Read the model definition and answer for the solid it produces. Units are mm, in the model's axes. Face numbers are marked on the shaded views. Round coordinates to 2 decimals unless told otherwise and drop trailing zeros. Write each loop counter-clockwise with the first axis right and the second up, starting at its lowest first coordinate (ties: lowest second). Pieces come first, ordered by that corner, then holes. Notation, with made-up numbers: (52.5, -20.5) - (65.5, -20.5) arc R38 cw to (65.5, 18.5) - close; hole circle Ø7 at (51, -40). An arc over 180 degrees is marked (long way). Use one line per item in the form item = value. Start each with the question number.
1) The part is cut by section A-A, the plane y = 326. Give the vertices of the cut face in (x, z) (3 decimals).
2) The part is cut by section C-C, the plane z = 211.5. Give the vertices of the cut face in (x, y) (3 decimals).
3) For a pull along X with two mould halves and no side action, classify the marked faces 1, 2 and 3 as released by +X, released by -X, zero draft, split by the parting line, or undercut.
4) Consider line 1 along X through (y, z) = (326, 202) (3 decimals); line 2 along Y through (x, z) = (172, 225) (3 decimals); line 3 along Z through (x, y) = (167.75, 326) (3 decimals). Determine where each line is inside the solid, lowest interval first. Write a range as from..to.
5) Each of these flat-tipped pins is pushed along its axis until it touches: pin 1 (1 mm diameter, centred on x = 172.5, y = 325, fed in from -Z); pin 2 (1.5 mm diameter, centred on y = 328.5, z = 221.5, fed in from -X); pin 3 (1.5 mm diameter, centred on x = 173.5, z = 220, fed in from +Y); pin 4 (2 mm diameter, centred on x = 175.5, y = 327, fed in from -Z) (3 decimals). Where does it stop, or does it pass through?
6) The part is cut by section B-B, the plane x = 165.5. Give the vertices of the cut face in (y, z) (3 decimals), plus the area to 3 significant figures.
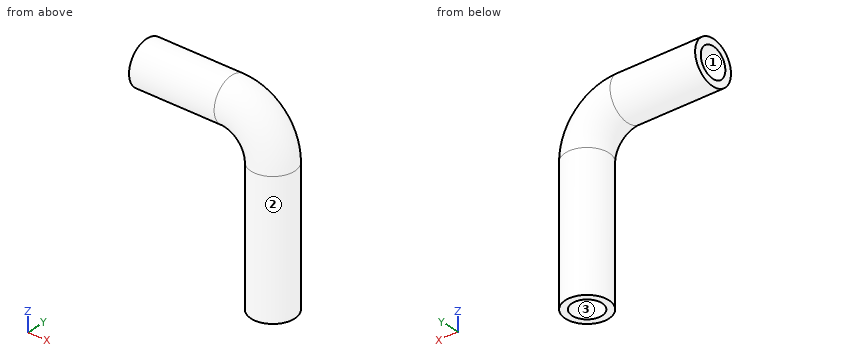
from build123d import *

# Parameters (mm, degrees)
TUBE_PROFILE_R   = 3.175
TUBE_PROFILE_R_2 = 2.175


with BuildPart() as part:
    # Tube: sweep along a curve in space
    with BuildLine() as tube_path:
        Line((182, 326, 199.5), (182, 326, 219))
        ThreePointArc((176, 326, 225), (180.242640687, 326, 223.242640687), (182, 326, 219))
        Line((176, 326, 225), (163.5, 326, 225))
    # Tube profile (on start of the path) → Tube (sweep)
    with BuildSketch(Plane(origin=(182, 326, 199.5), x_dir=(1, 0, 0), z_dir=(0, 0, 1))):
        Circle(TUBE_PROFILE_R)
        Circle(TUBE_PROFILE_R_2, mode=Mode.SUBTRACT)
    sweep(path=tube_path.line)


solid = part.part
Geometry results:
q1.outline = (163.5, 221.825) - (176, 221.825) arc R2.825 cw to (178.825, 219) - (178.825, 199.5) - (179.825, 199.5) - (179.825, 219) arc R3.825 ccw to (176, 222.825) - (163.5, 222.825) - close; (163.5, 227.175) - (176, 227.175) arc R8.175 cw to (184.175, 219) - (184.175, 199.5) - (185.175, 199.5) - (185.175, 219) arc R9.175 ccw to (176, 228.175) - (163.5, 228.175) - close
q2.outline = circle Ø6.35 at (182, 326); hole circle Ø4.35 at (182, 326)
q3.face_1 = zero draft
q3.face_2 = split by the parting line
q3.face_3 = undercut
q4.line_1 = 178.825..179.825, 184.175..185.175
q4.line_2 = 322.825..323.825, 328.175..329.175
q4.line_3 = 221.825..222.825, 227.175..228.175
q5.pin_1 = 221.86
q5.pin_2 = 177.77
q5.pin_3 = through
q5.pin_4 = 221.825
q6.outline = circle Ø6.35 at (326, 225); hole circle Ø4.35 at (326, 225)
q6.area = 16.8 mm2
